from build123d import *

# Parameters (mm, degrees)
F1_DEPTH = 8
F2_R     = 1.5
F3_DEPTH = 25
F4_R     = 3


# Not quite as in the source:
# - a pattern or mirror of a feature is missing from the dataset's text; its kind, count and spacing are read off the source's solid


with BuildPart() as f1:
    # F0 (on Front) → F1 (new body)
    with BuildSketch(Plane.XZ):
        with BuildLine():
            Line((11, 0), (11, 8.05))
            Line((11, 8.05), (4.95, 8.05))
            ThreePointArc((4.95, 8.05), (3.1978508408, 5.141515639), (0, 4))
            Line((0, 4), (0, 0))
            Line((0, 0), (11, 0))
        make_face()
    extrude(amount=F1_DEPTH)

    # F1_copies: F1 across plane


with BuildPart() as f1_1:
    add(f1.part)
    add(f1.part.mirror(Plane(origin=(0, 0, 0), x_dir=(0, 0, -1), z_dir=(-1, 0, 0))))

    # F2 (on face) → F3 (cut)
    with BuildSketch(Plane.XY.offset(8.05)):
        with Locations((7.5, -4)):
            Circle(F2_R)
    f3 = extrude(amount=-F3_DEPTH, mode=Mode.SUBTRACT)

    # F3_copies: F3 across plane
    add(f3.mirror(Plane(origin=(0, 0, 0), x_dir=(0, 0, -1), z_dir=(-1, 0, 0))), mode=Mode.SUBTRACT)

    # F4
    f4_edges = [f1_1.edges().sort_by_distance(p)[0] for p in [
        (11, 0, 4.025),
        (11, -8, 4.025),
        (-11, 0, 4.025),
        (-11, -8, 4.025),
    ]]
    fillet(f4_edges, radius=F4_R)


solid = f1_1.part
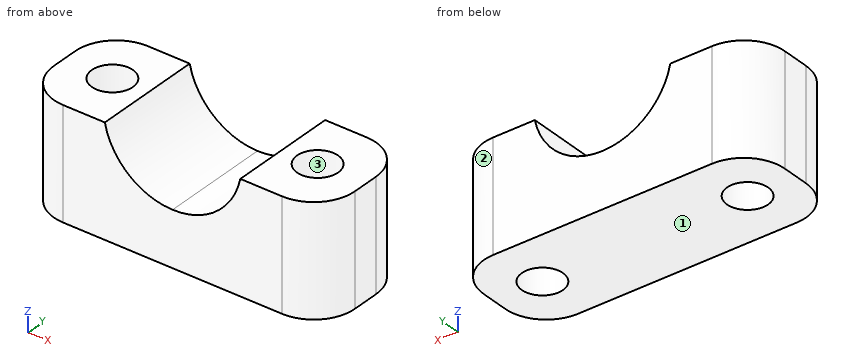
Can you work these out from the model? Positions are in its coordinate system, mm. Face numbers are marked on the shaded views. Round coordinates to 2 decimals unless told otherwise and drop trailing zeros. Write each loop counter-clockwise with the first axis right and the second up, starting at its lowest first coordinate (ties: lowest second). Pieces come first, ordered by that corner, then holes. Notation, with made-up numbers: (15.25, 34) - (30.25, 34) arc R14 ccw to (30.25, 43) - close; hole circle Ø9 at (77.5, -40). An arc over 180 degrees is marked (long way). Write each question's results on one line, items separated by ' | '. Start each with the question number.
1) Suppose I cut it at C-C (x = -7.5). List the corners of the cut face in (y, z) for me.
2) Suppose I cut it at B-B (z = 3.25). List the corners of the cut face in (x, y) for me, and give its area (3 significant figures).
3) We'd pull the mould along Y, two halves only. Please class the marked faces 1, 2 and 3: released by +Y, released by -Y, zero draft, split by the parting line, or undercut.
4) For pin 1 Ø1.8 at (x, y) = (-7.5, -4) entering from +Z, with a flat end and sliding along its axis, tell me the tip position at first contact or that it passes through.
5) Please list where these lines run through material, in increasing order: line 1 (Y direction, x = -7.5, z = 2.25); line 2 (X direction, y = -3.75, z = 3); line 3 (X direction, y = -5.25, z = 6.75).
6) Suppose I cut it at A-A (y = -4). List the corners of the cut face in (x, z) for me, and give its area (3 significant figures).
7) Suppose I cut it at D-D (z = 7). List the corners of the cut face in (x, y) for me, and give its area (3 significant figures).
Here are the results:
1) outline: (-8, 0) - (-5.5, 0) - (-5.5, 8.05) - (-8, 8.05) - close; (-2.5, 0) - (0, 0) - (0, 8.05) - (-2.5, 8.05) - close
2) outline: (-11, -5) arc R3 ccw to (-8, -8) - (8, -8) arc R3 ccw to (11, -5) - (11, -3) arc R3 ccw to (8, 0) - (-8, 0) arc R3 ccw to (-11, -3) - close; hole circle Ø3 at (-7.5, -4); hole circle Ø3 at (7.5, -4) | area: 154 mm2
3) face 1: zero draft | face 2: released by +Y | face 3: undercut
4) pin 1: passes through
5) line 1: y = -8 to -5.5, -2.5 to 0 | line 2: x = -11 to -8.98, -6.02 to 6.02, 8.98 to 11 | line 3: x = -10.99 to -8.33, -6.67 to -4.5, 4.5 to 6.67, 8.33 to 10.99
6) outline: (-11, 0) - (-9, 0) - (-9, 8.05) - (-11, 8.05) - close; (-6, 0) - (6, 0) - (6, 8.05) - (4.95, 8.05) arc R5.05 cw to (-4.95, 8.05) - (-6, 8.05) - close; (9, 0) - (11, 0) - (11, 8.05) - (9, 8.05) - close | area: 98.8 mm2
7) outline: (-11, -5) arc R3 ccw to (-8, -8) - (-4.62, -8) - (-4.62, 0) - (-8, 0) arc R3 ccw to (-11, -3) - close; (4.62, -8) - (8, -8) arc R3 ccw to (11, -5) - (11, -3) arc R3 ccw to (8, 0) - (4.62, 0) - close; hole circle Ø3 at (-7.5, -4); hole circle Ø3 at (7.5, -4) | area: 80.3 mm2
